```python
from build123d import *

# Parameters (mm, degrees)
SKETCH1_W           = 140
SKETCH1_H           = 50
BOSS_EXTRUDE1_DEPTH = 3
SKETCH2_R           = 1.6
CUT_EXTRUDE1_DEPTH  = 3
SKETCH3_R           = 12
CUT_EXTRUDE2_DEPTH  = 3
CHAMFER1_SIZE       = 1
CHAMFER2_SIZE       = 3
SKETCH4_R           = 3
SKETCH4_R_2         = 1.45
BOSS_EXTRUDE2_DEPTH = 13
FILLET1_R           = 2
SKETCH5_W           = 12.2
SKETCH5_H           = 14
CUT_EXTRUDE3_DEPTH  = 13
SKETCH6_W           = 3
SKETCH6_H           = 7
BOSS_EXTRUDE3_DEPTH = 2
SKETCH7_W           = 18.2
SKETCH7_H           = 7
BOSS_EXTRUDE4_DEPTH = 2


with BuildPart() as part:
    # Sketch1 → Boss-Extrude1 (new body)
    with BuildSketch(Plane(origin=(0, 0, 0), x_dir=(1, 0, 0), z_dir=(0, 1, 0))):
        with Locations((25.027932961, -7.332402235)):
            Rectangle(SKETCH1_W, SKETCH1_H)
    extrude(amount=BOSS_EXTRUDE1_DEPTH)

    # Sketch2 → Cut-Extrude1 (cut)
    with BuildSketch(Plane(origin=(0, 3, 0), x_dir=(1, 0, 0), z_dir=(0, 1, 0))):
        with Locations(Location((-41.972067039, 14.667597765, 0), (0, 0, 270))):
            Circle(SKETCH2_R)
        with Locations(Location((92.027932961, 14.667597765, 0), (0, 0, 270))):
            Circle(SKETCH2_R)
        with Locations(Location((-41.972067039, -29.332402235, 0), (0, 0, 270))):
            Circle(SKETCH2_R)
        with Locations(Location((92.027932961, -29.332402235, 0), (0, 0, 270))):
            Circle(SKETCH2_R)
    extrude(amount=-CUT_EXTRUDE1_DEPTH, mode=Mode.SUBTRACT)

    # Sketch3 → Cut-Extrude2 (cut)
    with BuildSketch(Plane(origin=(0, 3, 0), x_dir=(1, 0, 0), z_dir=(0, 1, 0))):
        with Locations(Location((35.027932961, -7.332402235, 0), (0, 0, 270))):
            Circle(SKETCH3_R)
    extrude(amount=-CUT_EXTRUDE2_DEPTH, mode=Mode.SUBTRACT)

    # Chamfer1
    chamfer1_edges = [part.edges().sort_by_distance(p)[0] for p in [
        (92.027932961, 3, -16.267597765),
        (-41.972067039, 3, 27.732402235),
        (92.027932961, 3, 27.732402235),
        (-41.972067039, 3, -16.267597765),
    ]]
    chamfer(chamfer1_edges, length=CHAMFER1_SIZE)

    # Chamfer2
    chamfer2_edges = [part.edges().sort_by_distance(p)[0] for p in [
        (35.027932961, 0, -4.667597765),
    ]]
    chamfer(chamfer2_edges, length=CHAMFER2_SIZE - 0.0001)  # a hair under: the kernel refuses the full size

    # Sketch4 → Boss-Extrude2 (add)
    # profile 1 of 4: a face of its own
    with BuildSketch(Plane.XZ):
        with Locations(Location((19.787932961, -7.907597765, 0), (0, 0, 90))):
            Circle(SKETCH4_R)
        with Locations(Location((19.787932961, -7.907597765, 0), (0, 0, 90))):
            Circle(SKETCH4_R_2, mode=Mode.SUBTRACT)
    # profile 2 of 4: a face of its own
    with BuildSketch(Plane.XZ):
        with Locations(Location((19.587932961, 22.572402235, 0), (0, 0, 90))):
            Circle(SKETCH4_R)
        with Locations(Location((19.587932961, 22.572402235, 0), (0, 0, 90))):
            Circle(SKETCH4_R_2, mode=Mode.SUBTRACT)
    # profile 3 of 4: a face of its own
    with BuildSketch(Plane.XZ):
        with Locations(Location((50.067932961, 22.772402235, 0), (0, 0, 90))):
            Circle(SKETCH4_R)
        with Locations(Location((50.067932961, 22.772402235, 0), (0, 0, 90))):
            Circle(SKETCH4_R_2, mode=Mode.SUBTRACT)
    # profile 4 of 4: a face of its own
    with BuildSketch(Plane.XZ):
        with Locations(Location((50.267932961, -7.707597765, 0), (0, 0, 90))):
            Circle(SKETCH4_R)
        with Locations(Location((50.267932961, -7.707597765, 0), (0, 0, 90))):
            Circle(SKETCH4_R_2, mode=Mode.SUBTRACT)
    extrude(amount=BOSS_EXTRUDE2_DEPTH)

    # Fillet1
    fillet1_edges = [part.edges().sort_by_distance(p)[0] for p in [
        (19.787932961, 0, -10.907597765),
        (19.587932961, 0, 19.572402235),
        (50.067932961, 0, 19.772402235),
        (50.267932961, 0, -10.707597765),
    ]]
    fillet(fillet1_edges, radius=FILLET1_R)

    # Sketch5 → Cut-Extrude3 (cut)
    with BuildSketch(Plane(origin=(0, 3, 0), x_dir=(1, 0, 0), z_dir=(0, 1, 0))):
        with Locations((-20.872067039, -7.332402235)):
            Rectangle(SKETCH5_W, SKETCH5_H)
        with Locations((3.327932961, -7.332402235)):
            Rectangle(SKETCH5_W, SKETCH5_H)
        with Locations((64.127932961, -7.332402235)):
            Rectangle(SKETCH5_W, SKETCH5_H)
    extrude(amount=-CUT_EXTRUDE3_DEPTH, mode=Mode.SUBTRACT)

    # Sketch6 → Boss-Extrude3 (add)
    with BuildSketch(Plane.XZ):
        with Locations((-28.472067039, 7.332402235)):
            Rectangle(SKETCH6_W, SKETCH6_H)
        with Locations((-13.272067039, 7.332402235)):
            Rectangle(SKETCH6_W, SKETCH6_H)
        with Locations((-4.272067039, 7.332402235)):
            Rectangle(SKETCH6_W, SKETCH6_H)
        with Locations((10.927932961, 7.332402235)):
            Rectangle(SKETCH6_W, SKETCH6_H)
        with Locations((56.527932961, 7.332402235)):
            Rectangle(SKETCH6_W, SKETCH6_H)
        with Locations((71.727932961, 7.332402235)):
            Rectangle(SKETCH6_W, SKETCH6_H)
    extrude(amount=BOSS_EXTRUDE3_DEPTH)

    # Sketch7 → Boss-Extrude4 (add)
    with BuildSketch(Plane.XZ.offset(2)):
        with Locations((-20.872067039, 7.332402235)):
            Rectangle(SKETCH7_W, SKETCH7_H)
        with Locations((3.327932961, 7.332402235)):
            Rectangle(SKETCH7_W, SKETCH7_H)
        with Locations((64.127932961, 7.332402235)):
            Rectangle(SKETCH7_W, SKETCH7_H)
    extrude(amount=BOSS_EXTRUDE4_DEPTH)


solid = part.part
```
Work out the finished part from the listing and answer in its coordinate system (mm). A direction names the side the tool comes from. Give positions to 0.01 mm unless a question says otherwise; leave off trailing zeros. Loops run counter-clockwise (first coordinate to the right, second up) from the corner with the lowest first, then second, coordinate; pieces in that order, holes last. Notation, with made-up numbers: (44.25, 77.5) -> (78.25, 77.5) arc R11 ccw to (78.25, 96.5) -> close; hole circle Ø2 at (71, 26.25). An arc over 180 degrees is marked (long way). One line per question, with ' | ' between items. Start each with the question number.
1) Straight lines are drawn through the part: L1, parallel to X at y = -10.5, z = 22; L2, parallel to X at y = 1.5, z = 2; L3, parallel to X at y = -8, z = -9. For each, find the intervals that lie inside material, in ascending order.
2) Section A-A, the plane x = 3 is taken. Determine the outline of the cut face in (y, z), then the cut area to 3 significant figures.
3) Each of these flat-tipped pins is pushed along its axis until it touches: pin 1 (4 mm diameter, centred on x = -28, z = 10, fed in from -Y); pin 2 (2 mm diameter, centred on x = 66, y = -3, fed in from -Z); pin 3 (4 mm diameter, centred on y = -4, z = 9, fed in from -X). Where does it stop, or does it pass through?
4) Section D-D, the plane x = 80 is taken. Determine the outline of the cut face in (y, z).
5) Section B-B, the plane y = -10 is taken. Determine the outline of the cut face in (x, z), then the cut area to 3 significant figures.
6) For faces 1 (the face through (-5.772, -2, 7)), 2 (the face through (3, 2, 14.332)), 3 (the face through (58.028, 1, 7)), determine the directions among +Z, -Z, +X, -X, +Y, -Y from which every point of the face is accessible in a straight line to the end or side of a thin tool.
7) Section C-C, the plane z = 29.5 is taken. State how many separate pieces and enclosed holes the cut face has, then the cut area to 3 significant figures.
8) Determine the mould class of faces 4 (the face through (24, 3, 1)), 5 (the face through (20, 0, 23)) for opening direction X: +X half, -X half, draft (parallel to the pull), parting line (faces both ways), or undercut.
Resolved:
1) L1: 16.64 to 18.26, 20.92 to 22.53, 47.17 to 48.84, 51.3 to 52.97 | L2: -44.97 to -26.97, -14.77 to -2.77, 9.43 to 22.63, 47.43 to 58.03, 70.23 to 95.03 | L3: 16.99 to 18.83, 20.74 to 22.58, 47.56 to 49.61, 50.93 to 52.98
2) outline: (-4, 3.83) -> (-2, 3.83) -> (-2, 10.83) -> (-4, 10.83) -> close; (0, -17.67) -> (3, -17.67) -> (3, 0.33) -> (0, 0.33) -> close; (0, 14.33) -> (3, 14.33) -> (3, 32.33) -> (0, 32.33) -> close | area: 122 mm2
3) pin 1: y = -4 | pin 2: z = 3.83 | pin 3: x = -29.97
4) outline: (0, -17.67) -> (3, -17.67) -> (3, 32.33) -> (0, 32.33) -> close
5) outline: circle Ø6 at (19.59, 22.57); circle Ø6 at (19.79, -7.91); circle Ø6 at (50.07, 22.77); circle Ø6 at (50.27, -7.71); hole circle Ø2.9 at (19.59, 22.57); hole circle Ø2.9 at (19.79, -7.91); hole circle Ø2.9 at (50.07, 22.77); hole circle Ø2.9 at (50.27, -7.71) | area: 86.7 mm2
6) face 1: +Z, -Z, -Y | face 2: +Y, -Y | face 3: +Y
7) separate pieces: 3 | enclosed holes: 0 | area: 399 mm2
8) face 4: draft | face 5: undercut
